```python
from build123d import *

# Parameters (mm, degrees)
SKETCH1_R           = 3.175
BOSS_EXTRUDE3_DEPTH = 3.96875
THREAD1_PITCH       = 1.058333333
SKETCH5_W           = 11.495261482
SKETCH5_H           = 9.373628012
CUT_EXTRUDE1_DEPTH  = 3.96875


with BuildPart() as part:
    # Sketch1 → Boss-Extrude3 (new body)
    with BuildSketch(Plane(origin=(0, 0, 0), x_dir=(1, 0, 0), z_dir=(0, 1, 0))):
        Polygon((-3.226233304, -5.588), (3.226233304, -5.588), (6.452466608, 0), (3.226233304, 5.588), (-3.226233304, 5.588), (-6.452466608, 0), align=None)
        with Locations(Location((0, 0, 0), (0, 0, 270))):
            Circle(SKETCH1_R, mode=Mode.SUBTRACT)
    extrude(amount=BOSS_EXTRUDE3_DEPTH)

    # Thread1: the profile of Thread Profile1 profile screwed along a right-hand helix of 3.75 turns, 8 arcs to a turn; built about Z, then put on its axis
    thread1_z = Axis((0, 0, 0), (0, 0, 1))
    thread1_corners = [(3.1753, 0, -0.000173205), (3.1753, 0, 0.926214869), (2.602160282, 0, 0.595312499), (2.602160282, 0, 0.330729165)]
    with BuildLine(mode=Mode.PRIVATE) as thread1_profile:
        Line(thread1_corners[0], thread1_corners[1])
        Line(thread1_corners[1], thread1_corners[2])
        Line(thread1_corners[2], thread1_corners[3])
        Line(thread1_corners[3], thread1_corners[0])
    thread1_cap = Face(thread1_profile.wire())
    thread1_turn_angles = [0, 22.5, 45, 67.5, 90, 112.5, 135, 157.5, 180, 202.5, 225, 247.5, 270, 292.5, 315, 337.5, 360]
    thread1_turn_weights = [1, 0.9238795325112867, 1, 0.9238795325112867, 1, 0.9238795325112867, 1, 0.9238795325112867, 1, 0.9238795325112867, 1, 0.9238795325112867, 1, 0.9238795325112867, 1, 0.9238795325112867, 1]
    thread1_turn_rails = [Edge.make_bspline([Vector(p[0], p[1], 0).rotate(thread1_z, thread1_turn_angles[k]) / thread1_turn_weights[k] + Vector(0, 0, p[2] + THREAD1_PITCH * thread1_turn_angles[k] / 360) for k in range(17)], [0, 0, 0, 1, 1, 2, 2, 3, 3, 4, 4, 5, 5, 6, 6, 7, 7, 8, 8, 8], 2, thread1_turn_weights) for p in thread1_corners]
    thread1_turn_sides = [Face.make_surface_from_curves(thread1_turn_rails[p[0]], thread1_turn_rails[p[1]]) for p in [(0, 1), (1, 2), (2, 3), (3, 0)]]
    thread1_last_angles = [1080, 1102.5, 1125, 1147.5, 1170, 1192.5, 1215, 1237.5, 1260, 1282.5, 1305, 1327.5, 1350]
    thread1_last_weights = [1, 0.9238795325112867, 1, 0.9238795325112867, 1, 0.9238795325112867, 1, 0.9238795325112867, 1, 0.9238795325112867, 1, 0.923879532511286, 1]
    thread1_last_rails = [Edge.make_bspline([Vector(p[0], p[1], 0).rotate(thread1_z, thread1_last_angles[k]) / thread1_last_weights[k] + Vector(0, 0, p[2] + THREAD1_PITCH * thread1_last_angles[k] / 360) for k in range(13)], [0, 0, 0, 1, 1, 2, 2, 3, 3, 4, 4, 5, 5, 6, 6, 6], 2, thread1_last_weights) for p in thread1_corners]
    thread1_last_sides = [Face.make_surface_from_curves(thread1_last_rails[p[0]], thread1_last_rails[p[1]]) for p in [(0, 1), (1, 2), (2, 3), (3, 0)]]
    thread1 = Plane(origin=(0, 3.96875, 0), x_dir=(-1, 0, 0), z_dir=(0, -1, 0)) * Solid(Shell([*[p.moved(Location((0, 0, THREAD1_PITCH * i))) for i in range(3) for p in thread1_turn_sides], *thread1_last_sides, thread1_cap, thread1_cap.rotate(thread1_z, 1350).moved(Location((0, 0, THREAD1_PITCH * 1350 / 360)))]))
    add(thread1)

    # Sketch5 → Cut-Extrude1 (cut)
    with BuildSketch(Plane(origin=(0, 0, 0), x_dir=(-1, 0, 0), z_dir=(0, -1, 0))):
        with Locations((0.048050932, -0.317875398)):
            Rectangle(SKETCH5_W, SKETCH5_H)
    extrude(amount=CUT_EXTRUDE1_DEPTH, mode=Mode.SUBTRACT)


solid = part.part
```
Model file for the job. Use its own axes, mm. Coordinates: 2 decimals unless noted, no trailing zeros. Loops run counter-clockwise (first coordinate to the right, second up) from the corner with the lowest first, then second, coordinate; pieces in that order, holes last. Notation, with made-up numbers: M 89,71.25 L 146,71.25 A21 cw 146,97.25 Z; hole C 65.25,80.5 d9. An arc over 180 degrees is marked long. Use CSV: the item, a comma, the result in double quotes. Start each with the question number.
1. Band-saw the part on A-A, the plane x = 3.5. List the corners of the cut face in (y, z).
2. Probe probe 1 along Z at (x, y) = (0, 1.65) (3 decimals); probe 2 along Z at (x, y) = (0, 0.9); probe 3 along X at (y, z) = (0.9, -1.25). List the from-to ranges inside material, lowest first. Write a range as [from, to].
3. Band-saw the part on B-B, the plane z = 4.5. List the corners of the cut face in (x, y).
Entries:
1,outline,"M 0,-5.11 L 3.97,-5.11 L 3.97,5.11 L 0,5.11 Z"
2,probe 1,"z = [-5.588, -3.175], [2.602, 5.588]"
2,probe 2,"z = [-5.59, -2.76], [2.9, 5.59]"
2,probe 3,"x = [-5.73, -2.84], [2.28, 5.73]"
3,outline,"M -3.85,0 L 3.85,0 L 3.85,3.97 L -3.85,3.97 Z"
